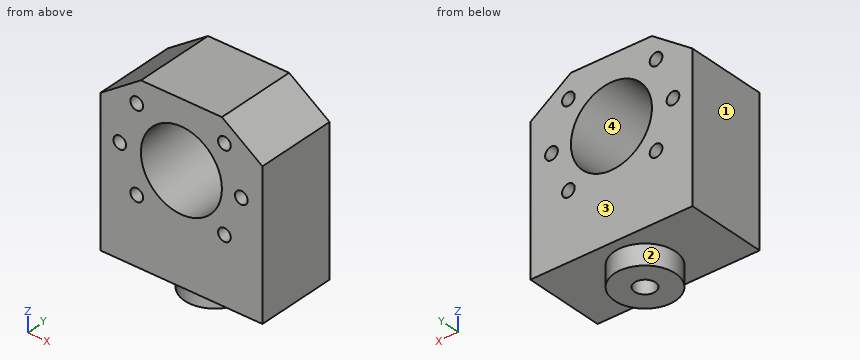
```python
from build123d import *

# Parameters (mm, degrees)
F0_W       = 50.8
F0_H       = 25.4
F1_DEPTH   = 27.178
F2_SIZE2   = 12.7
F2_SIZE    = 8.89
F2_2_SIZE2 = 12.7
F2_2_SIZE  = 8.89
F4_R       = 1.9939
F5_DEPTH   = 25.401
F3_R       = 12.7
F6_DEPTH   = 25.401
F7_R       = 9.5204472643
F8_DEPTH   = 6.35
F9_R       = 3.2639
F10_DEPTH  = 12.7


with BuildPart() as f1:
    # F0 (on Top) → F1 (new body, symmetric)
    with BuildSketch(Plane.XY):
        Rectangle(F0_W, F0_H)
    extrude(amount=F1_DEPTH, both=True)

    # F2
    f2_edges = [f1.edges().sort_by_distance(p)[0] for p in [
        (-25.4, 0, 27.178),
    ]]
    f2_side = f1.faces().sort_by_distance((-25.4, 0, 0))[0]
    chamfer(f2_edges, length=F2_SIZE, length2=F2_SIZE2, reference=f2_side)

    # F2#2
    f2_2_edges = [f1.edges().sort_by_distance(p)[0] for p in [
        (25.4, 0, 27.178),
    ]]
    f2_2_side = f1.faces().sort_by_distance((25.4, 0, 0))[0]
    chamfer(f2_2_edges, length=F2_2_SIZE, length2=F2_2_SIZE2, reference=f2_2_side)

    # F4 (on face) → F5 (cut, through all)
    with BuildSketch(Plane.XZ.offset(12.7)):
        with Locations((-14.0012001136, 19.9476279852)):
            Circle(F4_R)
        with Locations((13.4866058279, 19.9476279852)):
            Circle(F4_R)
        with Locations((18.7927028571, 6.477)):
            Circle(F4_R)
        with Locations((13.4866058279, -6.4347624395)):
            Circle(F4_R)
        with Locations((-14.0012001136, -6.4347624395)):
            Circle(F4_R)
        with Locations((-19.3072971429, 6.477)):
            Circle(F4_R)
    extrude(amount=-F5_DEPTH, mode=Mode.SUBTRACT)

    # F3 (on face) → F6 (cut, through all)
    with BuildSketch(Plane.XZ.offset(12.7)):
        with Locations((0, 6.477)):
            Circle(F3_R)
    extrude(amount=-F6_DEPTH, mode=Mode.SUBTRACT)

    # F7 (on face) → F8 (join)
    with BuildSketch(Plane(origin=(0, 0, -27.178), x_dir=(1, 0, 0), z_dir=(0, 0, -1))):
        Circle(F7_R)
    extrude(amount=F8_DEPTH)

    # F9 (on face) → F10 (cut)
    with BuildSketch(Plane(origin=(0, 0, -33.528), x_dir=(1, 0, 0), z_dir=(0, 0, -1))):
        Circle(F9_R)
    extrude(amount=-F10_DEPTH, mode=Mode.SUBTRACT)


solid = f1.part
```
The model under review builds one solid part; all positions refer to its coordinate system, in mm. Face numbers are marked on the shaded views. Coordinates: 2 decimals unless noted, no trailing zeros. Write each loop counter-clockwise with the first axis right and the second up, starting at its lowest first coordinate (ties: lowest second). Pieces come first, ordered by that corner, then holes. Notation, with made-up numbers: (84, -31.75) -> (91, -31.75) arc R20 cw to (91, 6.25) -> close; hole circle Ø1 at (-13.75, -22). An arc over 180 degrees is marked (long way). One line per item, written item: value. Start each with the question number.
Q1. To check wall thickness, follow probe 1 along Z at (x, y) = (0, -6.25); probe 2 along Z at (x, y) = (-3, -7); probe 3 along X at (y, z) = (6, -3.5). State the ranges of each line that lie inside material, in increasing order.
Q2. Add section B-B, the plane z = -26. Give the boundary of the cut face in (x, y), then the cut area to 3 significant figures.
Q3. The part is to be moulded in two halves that separate along X. For the marked faces 1, 2, 3 and 4, say which applies: +X half, -X half, draft (parallel to the pull), parting line (faces both ways), or undercut.
Q4. Clearance check with flat-ended pins moving along their axes: P1, Ø2, axis at x = 17, y = 2.5, coming from the +Z side; P2, Ø3.5, axis at x = 1, y = -0.5, coming from the -Z side. State where each tip first meets the part, or that it passes through.
Q5. Add section A-A, the plane x = 0. Give the boundary of the cut face in (y, z), then the cut area to 3 significant figures.
Q6. Add section C-C, the plane y = -7.5. Give the boundary of the cut face in (x, z), then the cut area to 3 significant figures.
Q7. Add section D-D, the plane z = 1.5. Give the boundary of the cut face in (x, y), then the cut area to 3 significant figures.
Response:
1. probe 1: -33.53 to -6.22, 19.18 to 27.18
1. probe 2: -33.53 to -5.86, 18.82 to 27.18
1. probe 3: -25.4 to -7.86, 7.86 to 25.4
2. outline: (-25.4, -12.7) -> (25.4, -12.7) -> (25.4, 12.7) -> (-25.4, 12.7) -> close; hole circle Ø6.53 at (0, 0)
2. area: 1,260 mm²
3. face 1: -X half
3. face 2: parting line
3. face 3: draft
3. face 4: undercut
4. P1: z = 24.87
4. P2: z = -20.83
5. outline: (-12.7, -27.18) -> (-9.52, -27.18) -> (-9.52, -33.53) -> (-3.26, -33.53) -> (-3.26, -20.83) -> (3.26, -20.83) -> (3.26, -33.53) -> (9.52, -33.53) -> (9.52, -27.18) -> (12.7, -27.18) -> (12.7, -6.22) -> (-12.7, -6.22) -> close; (-12.7, 19.18) -> (12.7, 19.18) -> (12.7, 27.18) -> (-12.7, 27.18) -> close
5. area: 773 mm²
6. outline: (-25.4, -27.18) -> (-5.86, -27.18) -> (-5.86, -33.53) -> (5.86, -33.53) -> (5.86, -27.18) -> (25.4, -27.18) -> (25.4, 18.29) -> (12.7, 27.18) -> (-12.7, 27.18) -> (-25.4, 18.29) -> close; hole circle Ø3.99 at (-19.31, 6.48); hole circle Ø3.99 at (-14, -6.43); hole circle Ø3.99 at (-14, 19.95); hole circle Ø25.4 at (0, 6.48); hole circle Ø3.99 at (13.49, -6.43); hole circle Ø3.99 at (13.49, 19.95); hole circle Ø3.99 at (18.79, 6.48)
6. area: 2,140 mm²
7. outline: (-25.4, -12.7) -> (-11.68, -12.7) -> (-11.68, 12.7) -> (-25.4, 12.7) -> close; (11.68, -12.7) -> (25.4, -12.7) -> (25.4, 12.7) -> (11.68, 12.7) -> close
7. area: 697 mm²
